Here's how the part is built. I have some questions about the finished solid (model axes, mm). A direction names the side the tool comes from. Round coordinates to 2 decimals unless told otherwise and drop trailing zeros. Loops run counter-clockwise (first coordinate to the right, second up) from the corner with the lowest first, then second, coordinate; pieces in that order, holes last. Notation, with made-up numbers: M 45.5,21.5 L 72.5,21.5 A22 cw 72.5,47.5 Z; hole C 18.5,15.25 d1. An arc over 180 degrees is marked long. Answer as a JSON object with one key per item and string values.
from build123d import *

# Parameters (mm, degrees)
F0_W     = 56.709073
F0_H     = 57.382157
F1_DEPTH = 25.4
F2_R     = 8.717495
F2_R_2   = 9.169361
F3_DEPTH = 25.4


with BuildPart() as f1:
    # F0 (on Front) → F1 (new body)
    with BuildSketch(Plane.XZ):
        with Locations((-28.354536, 3.497539)):
            Rectangle(F0_W, F0_H)
    extrude(amount=F1_DEPTH)

    # F2 (on Front) → F3 (join)
    with BuildSketch(Plane.XZ):
        with Locations((-56.388002, -25.4508)):
            Circle(F2_R)
        with Locations((0, -25.146002)):
            Circle(F2_R_2)
    extrude(amount=F3_DEPTH)


solid = f1.part
Item 1: For faces 1 (the face through (-62.55, -12.52, -31.62)), 2 (the face through (0, -13, 8)), 3 (the face through (-56.709, -13, 7)), 4 (the face through (-29, -13, 32.189)), 5 (the face through (-29, -13, -25.194)), which set-ups out of +Z, -Z, +X, -X, +Y, -Y let a thin tool reach every point of the face, with its end or its side?
Solution:
{"face 1": "+Y, -Y", "face 2": "+Z, +X, +Y, -Y", "face 3": "+Z, -X, +Y, -Y", "face 4": "+Z, +X, -X, +Y, -Y", "face 5": "-Z, +Y, -Y"}
Item 2: I want a section at D-D on z = -4. List the corners of the cut face in (x, y) for me.
Solution:
{"outline": "M -56.71,-25.4 L 0,-25.4 L 0,0 L -56.71,0 Z"}
Item 3: I want a section at C-C on x = -38.5. List the corners of the cut face in (y, z) for me.
Solution:
{"outline": "M -25.4,-25.19 L 0,-25.19 L 0,32.19 L -25.4,32.19 Z"}
Item 4: I want a section at B-B on z = -28. List the corners of the cut face in (x, y) for me, plus the area to 3 significant figures.
Solution:
{"outline": "M -64.72,-25.4 L -48.05,-25.4 L -48.05,0 L -64.72,0 Z; M -8.71,-25.4 L 8.71,-25.4 L 8.71,0 L -8.71,0 Z", "area": "866 mm2"}
Item 5: For P1, Ø5, axis at x = -21.5, z = -26, coming from the +Y side; P2, Ø1.5, axis at y = -4, z = 16.5, coming from the -X side; P3, Ø7.5, axis at y = -13, z = 15, coming from the +X side; P4, Ø1.5, axis at x = -37.5, y = -10, coming from the -Z side, each with a flat end and sliding along its axis, tell me the tip position at first contact or that it passes through.
Solution:
{"P1": "stops at y = 0", "P2": "stops at x = -56.71", "P3": "stops at x = 0", "P4": "stops at z = -25.19"}
Item 6: I want a section at A-A on y = -5.75. List the corners of the cut face in (x, z) for me, plus the area to 3 significant figures.
Solution:
{"outline": "M -56.71,-16.74 A8.72 ccw long -47.67,-25.19 L -9.17,-25.19 A9.17 ccw long 0,-15.98 L 0,32.19 L -56.71,32.19 Z", "area": "3,630 mm2"}
Item 7: If I drill on L1, parallel to X at y = -18, z = 11.5; L2, parallel to Z at x = -25, y = -20.5; L3, parallel to X at y = -20, z = -28.5, over which ranges is the centre line in solid material (lowest first)? Write a range as from..to.
Solution:
{"L1": "x = -56.71..0", "L2": "z = -25.19..32.19", "L3": "x = -64.55..-48.22, -8.53..8.53"}
